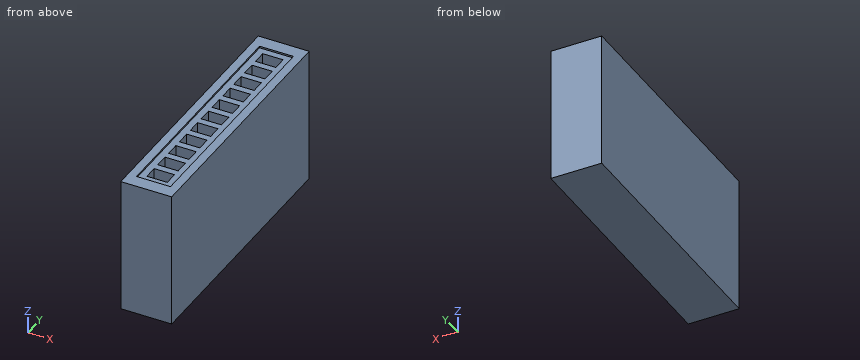
```python
from build123d import *

# Parameters (mm, degrees)
F0_W     = 0.4
F0_H     = 0.8
F0_W_2   = 1.2
F1_DEPTH = 8
F0_H_2   = 0.4
F2_DEPTH = 7.9
F3_DEPTH = 0.1


with BuildPart() as f1:
    # F0 (on Top) → F1 (new body)
    with BuildSketch(Plane.XY):
        with Locations((-119.9873028874, 4.3633364267)):
            Rectangle(F0_W, F0_H)
        Polygon((-120.6873028874, 19.1633364267), (-120.6873028874, 3.9633364267), (-120.1873028874, 3.9633364267), (-120.1873028874, 4.7633364267), (-120.1873028874, 5.1633364267), (-120.1873028874, 5.9633364267), (-120.1873028874, 6.3633364267), (-120.1873028874, 7.1633364267), (-120.1873028874, 7.5633364267), (-120.1873028874, 8.3633364267), (-120.1873028874, 8.7633364267), (-120.1873028874, 9.5633364267), (-120.1873028874, 9.9633364267), (-120.1873028874, 10.7633364267), (-120.1873028874, 11.1633364267), (-120.1873028874, 11.9633364267), (-120.1873028874, 12.3633364267), (-120.1873028874, 13.1633364267), (-120.1873028874, 13.5633364267), (-120.1873028874, 14.3633364267), (-120.1873028874, 14.7633364267), (-120.1873028874, 15.5633364267), (-120.1873028874, 15.9633364267), (-120.1873028874, 16.7633364267), (-120.1873028874, 17.1633364267), (-120.1873028874, 17.9633364267), (-120.1873028874, 18.3633364267), (-120.1873028874, 19.1633364267), align=None)
        with Locations((-119.1873028874, 4.3633364267)):
            Rectangle(F0_W_2, F0_H)
        with Locations((-118.3873028874, 4.3633364267)):
            Rectangle(F0_W, F0_H)
        with Locations((-119.9873028874, 18.7633364267)):
            Rectangle(F0_W, F0_H)
        with Locations((-119.1873028874, 18.7633364267)):
            Rectangle(F0_W_2, F0_H)
        with Locations((-118.3873028874, 18.7633364267)):
            Rectangle(F0_W, F0_H)
        Polygon((-118.1873028874, 4.7633364267), (-118.1873028874, 3.9633364267), (-117.6873028874, 3.9633364267), (-117.6873028874, 19.1633364267), (-118.1873028874, 19.1633364267), (-118.1873028874, 18.3633364267), (-118.1873028874, 17.9633364267), (-118.1873028874, 17.1633364267), (-118.1873028874, 16.7633364267), (-118.1873028874, 15.9633364267), (-118.1873028874, 15.5633364267), (-118.1873028874, 14.7633364267), (-118.1873028874, 14.3633364267), (-118.1873028874, 13.5633364267), (-118.1873028874, 13.1633364267), (-118.1873028874, 12.3633364267), (-118.1873028874, 11.9633364267), (-118.1873028874, 11.1633364267), (-118.1873028874, 10.7633364267), (-118.1873028874, 9.9633364267), (-118.1873028874, 9.5633364267), (-118.1873028874, 8.7633364267), (-118.1873028874, 8.3633364267), (-118.1873028874, 7.5633364267), (-118.1873028874, 7.1633364267), (-118.1873028874, 6.3633364267), (-118.1873028874, 5.9633364267), (-118.1873028874, 5.1633364267), align=None)
    extrude(amount=F1_DEPTH)

    # F0 (on Top) → F2 (join)
    with BuildSketch(Plane.XY):
        with Locations((-119.9873028874, 4.9633364267)):
            Rectangle(F0_W, F0_H_2)
        with Locations((-119.1873028874, 4.9633364267)):
            Rectangle(F0_W_2, F0_H_2)
        with Locations((-118.3873028874, 4.9633364267)):
            Rectangle(F0_W, F0_H_2)
        with Locations((-118.3873028874, 5.5633364267)):
            Rectangle(F0_W, F0_H)
        with Locations((-118.3873028874, 6.1633364267)):
            Rectangle(F0_W, F0_H_2)
        with Locations((-119.1873028874, 6.1633364267)):
            Rectangle(F0_W_2, F0_H_2)
        with Locations((-119.9873028874, 6.1633364267)):
            Rectangle(F0_W, F0_H_2)
        with Locations((-119.9873028874, 5.5633364267)):
            Rectangle(F0_W, F0_H)
        with Locations((-119.9873028874, 6.7633364267)):
            Rectangle(F0_W, F0_H)
        with Locations((-119.9873028874, 8.5633364267)):
            Rectangle(F0_W, F0_H_2)
        with Locations((-119.9873028874, 9.1633364267)):
            Rectangle(F0_W, F0_H)
        with Locations((-119.9873028874, 9.7633364267)):
            Rectangle(F0_W, F0_H_2)
        with Locations((-119.9873028874, 10.3633364267)):
            Rectangle(F0_W, F0_H)
        with Locations((-119.9873028874, 11.5633364267)):
            Rectangle(F0_W, F0_H)
        with Locations((-119.9873028874, 12.7633364267)):
            Rectangle(F0_W, F0_H)
        with Locations((-119.9873028874, 13.3633364267)):
            Rectangle(F0_W, F0_H_2)
        with Locations((-119.9873028874, 14.5633364267)):
            Rectangle(F0_W, F0_H_2)
        with Locations((-119.9873028874, 15.1633364267)):
            Rectangle(F0_W, F0_H)
        with Locations((-119.9873028874, 15.7633364267)):
            Rectangle(F0_W, F0_H_2)
        with Locations((-119.9873028874, 16.3633364267)):
            Rectangle(F0_W, F0_H)
        with Locations((-119.9873028874, 16.9633364267)):
            Rectangle(F0_W, F0_H_2)
        with Locations((-119.9873028874, 17.5633364267)):
            Rectangle(F0_W, F0_H)
        with Locations((-119.9873028874, 18.1633364267)):
            Rectangle(F0_W, F0_H_2)
        with Locations((-119.1873028874, 18.1633364267)):
            Rectangle(F0_W_2, F0_H_2)
        with Locations((-118.3873028874, 18.1633364267)):
            Rectangle(F0_W, F0_H_2)
        with Locations((-118.3873028874, 17.5633364267)):
            Rectangle(F0_W, F0_H)
        with Locations((-118.3873028874, 16.9633364267)):
            Rectangle(F0_W, F0_H_2)
        with Locations((-118.3873028874, 16.3633364267)):
            Rectangle(F0_W, F0_H)
        with Locations((-118.3873028874, 15.7633364267)):
            Rectangle(F0_W, F0_H_2)
        with Locations((-118.3873028874, 15.1633364267)):
            Rectangle(F0_W, F0_H)
        with Locations((-118.3873028874, 13.9633364267)):
            Rectangle(F0_W, F0_H)
        with Locations((-118.3873028874, 14.5633364267)):
            Rectangle(F0_W, F0_H_2)
        with Locations((-118.3873028874, 11.5633364267)):
            Rectangle(F0_W, F0_H)
        with Locations((-118.3873028874, 10.9633364267)):
            Rectangle(F0_W, F0_H_2)
        with Locations((-118.3873028874, 10.3633364267)):
            Rectangle(F0_W, F0_H)
        with Locations((-118.3873028874, 8.5633364267)):
            Rectangle(F0_W, F0_H_2)
        with Locations((-118.3873028874, 7.9633364267)):
            Rectangle(F0_W, F0_H)
        with Locations((-118.3873028874, 7.3633364267)):
            Rectangle(F0_W, F0_H_2)
        with Locations((-118.3873028874, 6.7633364267)):
            Rectangle(F0_W, F0_H)
        with Locations((-119.9873028874, 7.3633364267)):
            Rectangle(F0_W, F0_H_2)
        with Locations((-119.9873028874, 10.9633364267)):
            Rectangle(F0_W, F0_H_2)
        with Locations((-119.9873028874, 12.1633364267)):
            Rectangle(F0_W, F0_H_2)
        with Locations((-119.9873028874, 13.9633364267)):
            Rectangle(F0_W, F0_H)
        with Locations((-119.9873028874, 7.9633364267)):
            Rectangle(F0_W, F0_H)
        with Locations((-119.1873028874, 16.9633364267)):
            Rectangle(F0_W_2, F0_H_2)
        with Locations((-119.1873028874, 15.7633364267)):
            Rectangle(F0_W_2, F0_H_2)
        with Locations((-119.1873028874, 14.5633364267)):
            Rectangle(F0_W_2, F0_H_2)
        with Locations((-119.1873028874, 13.3633364267)):
            Rectangle(F0_W_2, F0_H_2)
        with Locations((-119.1873028874, 12.1633364267)):
            Rectangle(F0_W_2, F0_H_2)
        with Locations((-119.1873028874, 10.9633364267)):
            Rectangle(F0_W_2, F0_H_2)
        with Locations((-119.1873028874, 9.7633364267)):
            Rectangle(F0_W_2, F0_H_2)
        with Locations((-119.1873028874, 8.5633364267)):
            Rectangle(F0_W_2, F0_H_2)
        with Locations((-119.1873028874, 7.3633364267)):
            Rectangle(F0_W_2, F0_H_2)
        with Locations((-118.3873028874, 9.1633364267)):
            Rectangle(F0_W, F0_H)
        with Locations((-118.3873028874, 9.7633364267)):
            Rectangle(F0_W, F0_H_2)
        with Locations((-118.3873028874, 12.1633364267)):
            Rectangle(F0_W, F0_H_2)
        with Locations((-118.3873028874, 12.7633364267)):
            Rectangle(F0_W, F0_H)
        with Locations((-118.3873028874, 13.3633364267)):
            Rectangle(F0_W, F0_H_2)
    extrude(amount=F2_DEPTH)

    # F0 (on Top) → F3 (join)
    with BuildSketch(Plane.XY):
        with Locations((-119.1873028874, 17.5633364267)):
            Rectangle(F0_W_2, F0_H)
        with Locations((-119.1873028874, 16.3633364267)):
            Rectangle(F0_W_2, F0_H)
        with Locations((-119.1873028874, 15.1633364267)):
            Rectangle(F0_W_2, F0_H)
        with Locations((-119.1873028874, 13.9633364267)):
            Rectangle(F0_W_2, F0_H)
        with Locations((-119.1873028874, 12.7633364267)):
            Rectangle(F0_W_2, F0_H)
        with Locations((-119.1873028874, 11.5633364267)):
            Rectangle(F0_W_2, F0_H)
        with Locations((-119.1873028874, 10.3633364267)):
            Rectangle(F0_W_2, F0_H)
        with Locations((-119.1873028874, 9.1633364267)):
            Rectangle(F0_W_2, F0_H)
        with Locations((-119.1873028874, 7.9633364267)):
            Rectangle(F0_W_2, F0_H)
        with Locations((-119.1873028874, 6.7633364267)):
            Rectangle(F0_W_2, F0_H)
        with Locations((-119.1873028874, 5.5633364267)):
            Rectangle(F0_W_2, F0_H)
    extrude(amount=F3_DEPTH)


solid = f1.part
```
Verification items for the finished model (mm, model axes). Coordinates: 2 decimals unless noted, no trailing zeros. Write each loop counter-clockwise with the first axis right and the second up, starting at its lowest first coordinate (ties: lowest second). Pieces come first, ordered by that corner, then holes. Notation, with made-up numbers: (-4, -7.5) - (31, -7.5) arc R20 cw to (31, 3.5) - close; hole circle Ø5 at (5, -1). An arc over 180 degrees is marked (long way). Write item = value, one per line.
Q1. Material ranges on L1, parallel to X at y = 14, z = 6; L2, parallel to Z at x = -119.3, y = 13.25, recorded low to high. Write a range as from..to.
Answer:
L1 = -120.69..-119.79, -118.59..-117.69
L2 = 0..7.9
Q2. Cross-section at A-A (y = 11.75). Enter the section's corners in (x, z), plus the area to 3 significant figures.
Answer:
outline = (-120.69, 0) - (-117.69, 0) - (-117.69, 8) - (-118.19, 8) - (-118.19, 7.9) - (-118.59, 7.9) - (-118.59, 0.1) - (-119.79, 0.1) - (-119.79, 7.9) - (-120.19, 7.9) - (-120.19, 8) - (-120.69, 8) - close
area = 14.4 mm²
Q3. Cross-section at B-B (z = 7). Give the number of separate pieces and of enclosed holes in the cut face, plus the area to 3 significant figures.
Answer:
separate_pieces = 1
enclosed_holes = 11
area = 35.0 mm²
